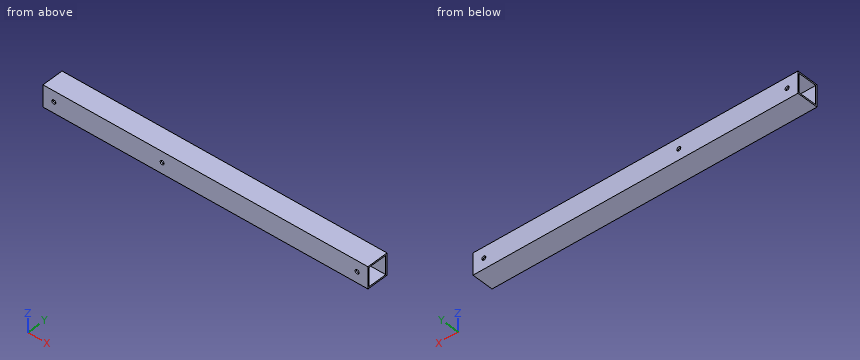
```python
from build123d import *

# Parameters (mm, degrees)
SKETCH1_W               = 30
SKETCH1_H               = 30
SKETCH1_W_2             = 26
SKETCH1_H_2             = 26
BOSS_EXTRUDE1_DEPTH     = 225
SKETCH2_R               = 2.75
CUT_EXTRUDE1_DEPTH      = 226.9977876
CUT_EXTRUDE2_DEPTH      = 226.9977876
CUT_EXTRUDE2_DEPTH_BACK = 226.9977876
SKETCH3_R               = 2.75


with BuildPart() as part:
    # Sketch1 → Boss-Extrude1 (new, symmetric)
    with BuildSketch(Plane(origin=(0, 0, 0), x_dir=(0, 0, -1), z_dir=(1, 0, 0))):
        Rectangle(SKETCH1_W, SKETCH1_H)
        Rectangle(SKETCH1_W_2, SKETCH1_H_2, mode=Mode.SUBTRACT)
    extrude(amount=BOSS_EXTRUDE1_DEPTH, both=True)

    # Sketch2 → Cut-Extrude1 (cut, symmetric)
    with BuildSketch(Plane(origin=(0, 0, 0), x_dir=(1, 0, 0), z_dir=(0, 1, 0))):
        with Locations(Location((210, 0, 0), (0, 0, 270))):
            Circle(SKETCH2_R)
    cut_extrude1 = extrude(amount=CUT_EXTRUDE1_DEPTH, both=True, mode=Mode.SUBTRACT)

    # Mirror1: Cut-Extrude1 across plane
    add(cut_extrude1.mirror(Plane(origin=(0, 0, 0), x_dir=(0, 0, 1), z_dir=(1, 0, 0))), mode=Mode.SUBTRACT)

    # Sketch3 → Cut-Extrude2 (cut, two sides: drawn at the far end of the back side and taken through both)
    with BuildSketch(Plane(origin=(0, 0, 0), x_dir=(1, 0, 0), z_dir=(0, 1, 0)).offset(-CUT_EXTRUDE2_DEPTH_BACK)):
        with Locations(Location((-60, 0, 0), (0, 0, 270))):
            Circle(SKETCH3_R)
    extrude(amount=CUT_EXTRUDE2_DEPTH + CUT_EXTRUDE2_DEPTH_BACK, mode=Mode.SUBTRACT)


solid = part.part
```
The listing builds one solid part. Answer for the finished solid, in the listing's coordinates (mm). Round coordinates to 2 decimals unless told otherwise and drop trailing zeros. Order: outer loops, then holes, each group sorted by start corner. A loop starts at its lowest first (then second) coordinate and runs counter-clockwise, first axis right, second up. Notation, with made-up numbers: (0, 75) - (33, 75) arc R35 cw to (33, 107) - close; hole circle Ø6 at (46, -10). An arc over 180 degrees is marked (long way). Put each result on its own line as item: value. Start each with the question number.
(1) Find section A-A (y = 2.5). Give the vertices of the cut face in (x, z).
(2) Given P1, Ø5, axis at x = -210, z = 0, coming from the -Y side, flat-ended and moving along its own axis, determine where the tip first touches the part or whether it passes through.
(3) Find section C-C (x = -148). Give the vertices of the cut face in (y, z).
(4) Straight lines are drawn through the part: probe 1 along X at (y, z) = (13.9, 0); probe 2 along Y at (x, z) = (72.5, -9.5). For each, find the intervals that lie inside material, in ascending order. Write a range as from..to.
Reply:
1. outline: (-225, -15) - (225, -15) - (225, -13) - (-225, -13) - close; (-225, 13) - (225, 13) - (225, 15) - (-225, 15) - close
2. P1: through
3. outline: (-15, -15) - (15, -15) - (15, 15) - (-15, 15) - close; hole (-13, -13) - (13, -13) - (13, 13) - (-13, 13) - close
4. probe 1: -225..-212.75, -207.25..-62.75, -57.25..207.25, 212.75..225
4. probe 2: -15..-13, 13..15
